Build history of the part. All positions in model axes, mm. A direction names the side the tool comes from. Round coordinates to 2 decimals unless told otherwise and drop trailing zeros.
from build123d import *

# Parameters (mm, degrees)
SKETCH1_W           = 100
SKETCH1_H           = 100
BOSS_EXTRUDE1_DEPTH = 12
BOSS_EXTRUDE2_DEPTH = 30
BOSS_EXTRUDE3_DEPTH = 8
BOSS_EXTRUDE4_DEPTH = 30
SKETCH8_W           = 100
SKETCH8_H           = 100
BOSS_EXTRUDE5_DEPTH = 12
SKETCH9_W           = 10
SKETCH9_H           = 10
BOSS_EXTRUDE6_DEPTH = 12
SKETCH19_R          = 1.25
CUT_EXTRUDE3_DEPTH  = 6
CUT_EXTRUDE4_START  = -6
SKETCH20_R          = 1.25
CUT_EXTRUDE4_DEPTH  = 6


with BuildPart() as part:
    # Sketch1 → Boss-Extrude1 (new body)
    with BuildSketch(Plane.XY):
        Rectangle(SKETCH1_W, SKETCH1_H)
        Polygon((-20, -38), (-20, -30.45), (20, -30.45), (20, -34.45), (34, -34.45), (34, 34.45), (20, 34.45), (20, 30.45), (-20, 30.45), (-20, 38), (-40, 38), (-40, 40), (40, 40), (40, -40), (-40, -40), (-40, -38), align=None, mode=Mode.SUBTRACT)
        Polygon((-20, -29.55), (-20, -22), (-40, -22), (-40, 22), (-20, 22), (-20, 29.55), (20, 29.55), (20, 15), (-15, 15), (-15, -15), (20, -15), (20, -29.55), align=None, mode=Mode.SUBTRACT)
    extrude(amount=BOSS_EXTRUDE1_DEPTH)

    # Sketch3 → Boss-Extrude2 (add)
    with BuildSketch(Plane.ZY.offset(15)):
        Polygon((14, 12.85), (14, 24.85), (0, 15), (12, 15), (12, -15), align=None)
    extrude(amount=-BOSS_EXTRUDE2_DEPTH)

    # Sketch4 → Boss-Extrude3 (add)
    with BuildSketch(Plane.XY.offset(14)):
        Polygon((-15, 12.85), (-15, 24.85), (-33.36063033, 24.85), (-36.135022811, 19.186760341), (-72.235731357, 36.872314969), (-70.475974677, 40.464425272), (-79.456250435, 44.863816971), (-87.810556524, 27.810556524), (-68, 8), (-68, 0), (-60, 0), (0, 0), (0, 8), (-49.718758429, 8), (-74.325442414, 32.606683984), (-72.565685734, 36.198794287), (-36.464977189, 18.513239659), (-39.23936967, 12.85), align=None)
        Polygon((15, 24.85), (15, 12.85), (39.23936967, 12.85), (36.464977189, 18.513239659), (72.565685734, 36.198794287), (74.325442414, 32.606683984), (49.718758429, 8), (0, 8), (0, 0), (60, 0), (68, 0), (68, 8), (87.810556524, 27.810556524), (79.456250435, 44.863816971), (70.475974677, 40.464425272), (72.235731357, 36.872314969), (36.135022811, 19.186760341), (33.36063033, 24.85), align=None)
        Polygon((6, 24.85), (0, 24.85), (0, 12.85), (15, 12.85), (15, 24.85), align=None)
        Polygon((0, 24.85), (-6, 24.85), (-15, 24.85), (-15, 12.85), (0, 12.85), align=None)
    boss_extrude3 = extrude(amount=BOSS_EXTRUDE3_DEPTH)

    # Mirror6: Boss-Extrude3 across plane
    add(boss_extrude3.mirror(Plane(origin=(0, 0, 22), x_dir=(0, 0, 1), z_dir=(0, 1, 0))))

    # Sketch7 → Boss-Extrude4 (add)
    with BuildSketch(Plane(origin=(15, 0, 0), x_dir=(0, -1, 0), z_dir=(-1, 0, 0))):
        Polygon((24.85, 22), (12.85, 22), (-15, 24), (15, 24), (15, 36), (24.85, 34), align=None)
    extrude(amount=BOSS_EXTRUDE4_DEPTH)

    # Sketch8 → Boss-Extrude5 (add)
    with BuildSketch(Plane.XY.offset(24)):
        Rectangle(SKETCH8_W, SKETCH8_H)
        Polygon((15, -15), (15, 20), (29.55, 20), (29.55, -20), (22, -20), (22, -40), (-22, -40), (-22, -20), (-29.55, -20), (-29.55, 20), (-15, 20), (-15, -15), align=None, mode=Mode.SUBTRACT)
        Polygon((38, -20), (30.45, -20), (30.45, 20), (34.45, 20), (34.45, 34), (-34.45, 34), (-34.45, 20), (-30.45, 20), (-30.45, -20), (-38, -20), (-38, -40), (-40, -40), (-40, 40), (40, 40), (40, -40), (38, -40), align=None, mode=Mode.SUBTRACT)
    extrude(amount=BOSS_EXTRUDE5_DEPTH)

    # Sketch9 → Boss-Extrude6 (add)
    with BuildSketch(Plane.XY.offset(12)):
        with Locations((35, -45)):
            Rectangle(SKETCH9_W, SKETCH9_H)
        with Locations((-35, -45)):
            Rectangle(SKETCH9_W, SKETCH9_H)
        with Locations((-35, 45)):
            Rectangle(SKETCH9_W, SKETCH9_H)
        with Locations((35, 45)):
            Rectangle(SKETCH9_W, SKETCH9_H)
    extrude(amount=BOSS_EXTRUDE6_DEPTH)

    # Sketch19 → Cut-Extrude3 (cut)
    with BuildSketch(Plane.XY.offset(36)):
        Circle(SKETCH19_R)
    extrude(amount=-CUT_EXTRUDE3_DEPTH, mode=Mode.SUBTRACT)

    # Sketch20 → Cut-Extrude4 (cut)
    with BuildSketch(Plane(origin=(0, 0, 0), x_dir=(-1, 0, 0), z_dir=(0, 0, -1)).offset(CUT_EXTRUDE4_START)):
        with Locations(Location((0, 0, 0), (0, 0, 180))):
            Circle(SKETCH20_R)
    extrude(amount=CUT_EXTRUDE4_DEPTH, mode=Mode.SUBTRACT)


solid = part.part
1) Which spindle directions (+Z, -Z, +X, -X, +Y, -Y) get a long thin tool onto all of the face, cutting with end or side? Do faces 4 (the flat face through (-1, 21, 24)), 5 (the flat face through (-37.833, 15.721, 17.944)), 6 (the flat face through (-15, 5, 7)). Say none if no direction does.
Results:
face 4: none
face 5: +Z, -Z
face 6: -Z
2) Wall check: L1, parallel to Y at x = 0, z = 33; L2, parallel to X at y = 0, z = 6.5; L3, parallel to X at y = -13.5, z = 29. Give the ranges that are in metal, low to high.
Results:
L1: y = -50 to -40, -24.85 to -1.25, 1.25 to 34, 40 to 50
L2: x = -50 to -40, -15 to 34, 40 to 50
L3: x = -50 to -40, -30.45 to -29.55, -15 to 15, 29.55 to 30.45, 40 to 50
3) Slice it at A-A (z = 27). Count the separate pieces of the cut face and the enclosed holes in it, plus the area to 3 significant figures.
Results:
separate pieces: 1
enclosed holes: 2
area: 6,620 mm2
4) Mould opens along Y. For faces 1 (the flat face through (18, 15, 6)), 2 (the flat face through (0, 45, 24)), 3 (the flat face through (-83.575, -36.457, 17.944)) say: released by +Y, released by -Y, zero draft, split by the parting line, or undercut.
Results:
face 1: undercut
face 2: zero draft
face 3: released by -Y
5) Pin check, flat tips, straight feed: pin 1 Ø3 at (y, z) = (22, 20) entering from +X; pin 2 Ø2 at (y, z) = (-11.5, 22) entering from +X; pin 3 Ø2 at (y, z) = (-31.5, 5) entering from -X; pin 4 Ø5 at (x, z) = (28.5, 17.5) entering from -Y. Stop position of each tip, or through.
Results:
pin 1: stops at x = 83.5
pin 2: stops at x = 72.5
pin 3: stops at x = -50
pin 4: stops at y = -50
